Part model, mm, in its own coordinate system. A direction names the side the tool comes from. Round coordinates to 2 decimals unless told otherwise and drop trailing zeros. Write each loop counter-clockwise with the first axis right and the second up, starting at its lowest first coordinate (ties: lowest second). Pieces come first, ordered by that corner, then holes. Notation, with made-up numbers: M 25.25,-10.75 L 75.25,-10.75 A25 cw 75.25,11.25 Z; hole C 9,-0.5 d7. An arc over 180 degrees is marked long. One line per question, with ' | ' between items. Start each with the question number.
1) Drop flat-ended pins along their axis: pin 1 Ø8 at (x, y) = (-6.5, 55.5) entering from +Z; pin 2 Ø2 at (y, z) = (31, 5) entering from +X; pin 3 Ø5 at (x, y) = (-8.09, 23.03) entering from -Z; pin 4 Ø4 at (x, y) = (17.5, 45) entering from +Z. Give the stop position or say it passes through.
2) Saw through at C-C (x = 19.36). List the corners of the cut face in (y, z), plus the area to 3 significant figures.
3) Mould opens along Y. For faces 1 (the face through (-8.5, 3.94, 5.07)), 2 (the face through (-7.308, 19.518, 1.479)), 3 (the face through (17.632, 35.993, 3.057)) say: pulls with the +Y half, pulls with the -Y half, needs draft (parallel to the pull), parting line crosses it, or undercut.
4) Wall check: probe 1 along Z at (x, y) = (6.18, 6.75); probe 2 along Z at (x, y) = (0, 20); probe 3 along X at (y, z) = (40.5, 4.75). Give the ranges that are in metal, low to high. Write a range as [from, to].
5) Saw through at A-A (x = 15). List the corners of the cut face in (y, z).
6) Tool access for faces 4 (the face through (-9, 26, 3)), 5 (the face through (19, 8, 5)), 6 (the face through (-11.82, 4.31, 8.77)): list every direction of +Z, -Z, +X, -X, +Y, -Y with a clear straight run to the whole face (end or side of a thin tool).
7) Saw through at B-B (x = -7.5). Give the number of separate pieces and of enclosed holes in the cut face, plus the area to 3 significant figures.
```python
from build123d import *

# Parameters (mm, degrees)
SKIZZE1_R                            = 2.1
AUFSATZ_LINEAR_AUSTRAGEN1_DEPTH      = 10
SKIZZE2_R                            = 1.5
SCHNITT_LINEAR_AUSTRAGEN1_DEPTH      = 8
SCHNITT_LINEAR_AUSTRAGEN3_DEPTH      = 2.8
SCHNITT_LINEAR_AUSTRAGEN5_DEPTH      = 69.862823313
SCHNITT_LINEAR_AUSTRAGEN5_DEPTH_BACK = 69.862823313
SKIZZE7_R                            = 10
FASE1_SIZE                           = 3
SCHNITT_LINEAR_AUSTRAGEN4_DEPTH      = 10
VERRUNDUNG1_R                        = 2
FASE2_SIZE                           = 1
FASE3_SIZE                           = 2.5
SKIZZE8_R                            = 3.6
SCHNITT_LINEAR_AUSTRAGEN6_DEPTH      = 3
FASE4_SIZE                           = 0.6


with BuildPart() as part:
    # Skizze1 → Aufsatz-Linear austragen1 (new body)
    with BuildSketch(Plane.XY):
        Polygon((28.287001282, 57.370618027), (28.287001282, 0), (-13.088781156, 0), (-13.088781156, 27.348243657), (-13.088781156, 53.715647777), (-13.088781156, 57.370618027), (-13.088781156, 62.370618027), (28.287001282, 62.370618027), align=None)
        with Locations((-8.088781156, 23.031945717)):
            Circle(SKIZZE1_R, mode=Mode.SUBTRACT)
        with Locations(Location((-8.088781156, 58.031945717, 0), (0, 0, 180))):
            Circle(SKIZZE1_R, mode=Mode.SUBTRACT)
    extrude(amount=AUFSATZ_LINEAR_AUSTRAGEN1_DEPTH)

    # Skizze2 → Schnitt-Linear austragen1 (cut)
    with BuildSketch(Plane.XZ):
        with Locations((-7, 5)):
            Circle(SKIZZE2_R)
        with Locations((6.18, 5)):
            Circle(SKIZZE2_R)
        with Locations((19.36, 5)):
            Circle(SKIZZE2_R)
    extrude(amount=-SCHNITT_LINEAR_AUSTRAGEN1_DEPTH, mode=Mode.SUBTRACT)

    # Skizze4 → Schnitt-Linear austragen3 (cut)
    with BuildSketch(Plane.XY.offset(10)):
        Polygon((-15.095168359, 10), (28.287001282, 10), (36.093332102, 46.989971623), (30.429094825, 65.957451721), (-16.081030445, 65.957451721), (-16.081030445, 27.753515123), align=None)
    extrude(amount=-SCHNITT_LINEAR_AUSTRAGEN3_DEPTH, mode=Mode.SUBTRACT)

    # Skizze7 → Schnitt-Linear austragen5 (cut, two sides: drawn at the far end of the back side and taken through both)
    with BuildSketch(Plane.XY.offset(7.2).offset(-SCHNITT_LINEAR_AUSTRAGEN5_DEPTH_BACK)):
        with Locations((-0.088781156, 40.531945717)):
            Circle(SKIZZE7_R)
    extrude(amount=SCHNITT_LINEAR_AUSTRAGEN5_DEPTH + SCHNITT_LINEAR_AUSTRAGEN5_DEPTH_BACK, mode=Mode.SUBTRACT)

    # Fase1
    # the kernel refuses this chamfer: 3 mm, written as the material it takes off along each edge
    with BuildSketch(Plane(origin=(-20.80383012, 10, 10), x_dir=(0, -0.9996219169112969, 0.027495876610586202), z_dir=(1, 0, 0))) as fase1_piece_1_section:
        Polygon((FASE1_SIZE * 0.999621916911, FASE1_SIZE * 0.0274958766106), (-FASE1_SIZE * 0.0274958766106, FASE1_SIZE * 0.999621916911), (0, 0), align=None)
    fase1_piece_1 = extrude(amount=56.805880365, mode=Mode.PRIVATE)
    fase1_piece_1 = split(fase1_piece_1, bisect_by=Plane(origin=(7.599110063, 8.999392985, 7.2), z_dir=(0, 0, 1)), keep=Keep.TOP, mode=Mode.PRIVATE)
    add(fase1_piece_1, mode=Mode.SUBTRACT)

    # Skizze5 → Schnitt-Linear austragen4 (cut)
    with BuildSketch(Plane(origin=(0, 0, 0), x_dir=(-1, 0, 0), z_dir=(0, 0, -1))):
        Polygon((-24.81273389, 11.736777957), (-9.824335871, 62.370618027), (-28.287001282, 62.370618027), (-28.287001282, 0), (-24.81273389, 0), align=None)
    extrude(amount=-SCHNITT_LINEAR_AUSTRAGEN4_DEPTH, mode=Mode.SUBTRACT)

    # Verrundung1
    verrundung1_edges = [part.edges().sort_by_distance(p)[0] for p in [
        (9.824335871, 62.370618027, 3.6),
        (-13.088781156, 62.370618027, 3.6),
    ]]
    fillet(verrundung1_edges, radius=VERRUNDUNG1_R)

    # Fase2
    fase2_edges = [part.edges().sort_by_distance(p)[0] for p in [
        (24.81273389, 10.768388979, 7.2),
        (24.81273389, 3.5, 10),
        (-13.088781156, 35.085309014, 7.2),
        (-1.379099888, 62.370618027, 7.2),
        (17.530529072, 36.337538735, 7.2),
        (9.527376482, 61.973016693, 7.2),
        (-12.502994718, 61.78483159, 7.2),
        (-10.088781156, 40.531945717, 7.2),
        (-13.088781156, 8.4, 8.6),
        (24.81273389, 8.4, 8.6),
    ]]
    chamfer(fase2_edges, length=FASE2_SIZE)

    # Fase3
    fase3_edges = [part.edges().sort_by_distance(p)[0] for p in [
        (-13.088781156, 2.792893219, 10),
    ]]
    chamfer(fase3_edges, length=FASE3_SIZE)

    # Skizze8 → Schnitt-Linear austragen6 (cut)
    with BuildSketch(Plane(origin=(0, 0, 0), x_dir=(-1, 0, 0), z_dir=(0, 0, -1))):
        with Locations((8.088781156, 23.031945717)):
            Circle(SKIZZE8_R)
    extrude(amount=-SCHNITT_LINEAR_AUSTRAGEN6_DEPTH, mode=Mode.SUBTRACT)

    # Fase4
    fase4_edges = [part.edges().sort_by_distance(p)[0] for p in [
        (-10.188781156, 23.031945717, 3),
    ]]
    chamfer(fase4_edges, length=FASE4_SIZE)


solid = part.part
```
Answer key:
1) pin 1: stops at z = 7.2 | pin 2: stops at x = 19.41 | pin 3: stops at z = 3.2 | pin 4: passes through
2) outline: M 0,0 L 30.16,0 L 30.16,6.2 L 26.63,7.2 L 9.8,7.2 L 7,10 L 0,10 L 0,6.5 L 8,6.5 L 8,3.5 L 0,3.5 Z | area: 215 mm2
3) face 1: needs draft | face 2: undercut | face 3: pulls with the +Y half
4) probe 1: z = [0, 3.5], [6.5, 10] | probe 2: z = [0, 7.2] | probe 3: x = [-13.09, -10.09], [9.91, 16.3]
5) outline: M 0,0 L 44.89,0 L 44.89,6.2 L 41.36,7.2 L 9.8,7.2 L 7,10 L 0,10 Z
6) face 4: -Z | face 5: -Y | face 6: +Z, -X, +Y, -Y
7) separate pieces: 4 | enclosed holes: 0 | area: 284 mm2
